Here's how the part is built. I have some questions about the finished solid (model axes, mm). Face numbers are marked on the shaded views. A direction names the side the tool comes from. Give positions to 0.01 mm unless a question says otherwise; leave off trailing zeros. Write each loop counter-clockwise with the first axis right and the second up, starting at its lowest first coordinate (ties: lowest second). Pieces come first, ordered by that corner, then holes. Notation, with made-up numbers: (39.5, 69) - (43.5, 69) arc R35 cw to (43.5, 107) - close; hole circle Ø10 at (11.5, 63.25). An arc over 180 degrees is marked (long way). One line per item, written item: value. Start each with the question number.
1) We'd pull the mould along X, two halves only. Please class the marked faces 4, 5 and 6: +X half, -X half, draft (parallel to the pull), parting line (faces both ways), or undercut.
2) Imagine slicing it at C-C on z = 32. Write out the boundary of the cut face in (x, y), plus the area to 3 significant figures.
3) Please list where these lines run through material, in increasing order: L1, parallel to X at y = 17, z = 4; L2, parallel to Y at x = 91.25, z = 19; L3, parallel to X at y = -4.5, z = 37. Write a range as [from, to].
4) On a 3-axis mill with a long thin cutter (end or side, diameter ignored), from which of +Z, -Z, +X, -X, +Y, -Y can I reach the whole of each face in a straight line? I mean the marked faces 1, 2 and 3. Say none if no direction works.
5) Imagine slicing it at A-A on z = 22. Write out the boundary of the cut face in (x, y), plus the area to 3 significant figures.
6) I'm going to push flat-ended pins straight in: P1, Ø1, axis at x = 97, y = 8, coming from the -Z side; P2, Ø8, axis at y = 8.5, z = 25.5, coming from the +X side (3 decimals); P3, Ø4, axis at y = -4, z = 35, coming from the +X side; P4, Ø1.5, axis at x = 108.8, z = 4, coming from the -Y side. Where does each tip first touch, or does it pass through?
7) Imagine slicing it at D-D on y = 5. Write out the boundary of the cut face in (x, z).
8) Imagine slicing it at B-B on x = 93.3. Write out the boundary of the cut face in (y, z).
from build123d import *

# Parameters (mm, degrees)
SKETCH_2_W          = 20
SKETCH_2_H          = 30
EXTRUDE_1_DEPTH     = 5
SKETCH_5_W          = 20
SKETCH_5_H          = 3
EXTRUDE_3_DEPTH     = 43.51
CUT_EXTRUDE_2_REACH = 125.027
SKETCH_6_W          = 5
SKETCH_6_H          = 13.035
EXTRUDE_4_DEPTH     = 3
CUT_EXTRUDE_3_REACH = 127.702
SKETCH_8_R          = 1.25
CUT_EXTRUDE_4_REACH = 127.702
SKETCH_9_R          = 1.25
CHAMFER_2_SIZE      = 8
CHAMFER_3_SIZE      = 11
EXTRUDE_6_DEPTH     = 3


with BuildPart() as part:
    # 草图2 → 凸台-拉伸1 (new body)
    with BuildSketch(Plane.XY.offset(38.51)):
        with Locations((99.3, 0)):
            Rectangle(SKETCH_2_W, SKETCH_2_H)
        with BuildLine():
            Line((104.3, -3.31662479), (104.3, 3.31662479))
            ThreePointArc((104.3, 3.31662479), (99.3, 6), (94.3, 3.31662479))
            Line((94.3, 3.31662479), (94.3, -3.31662479))
            ThreePointArc((94.3, -3.31662479), (99.3, -6), (104.3, -3.31662479))
        make_face(mode=Mode.SUBTRACT)
    extrude(amount=EXTRUDE_1_DEPTH)

    # 草图5 → 凸台-拉伸3 (add)
    with BuildSketch(Plane.XY.offset(43.51)):
        with Locations((99.3, 16.5)):
            Rectangle(SKETCH_5_W, SKETCH_5_H)
        with Locations((99.3, -16.5)):
            Rectangle(SKETCH_5_W, SKETCH_5_H)
    extrude(amount=-EXTRUDE_3_DEPTH)

    # 草图6 → 切除-拉伸2 (cut, up to next)
    with BuildSketch(Plane.XZ.offset(18), mode=Mode.PRIVATE) as cut_extrude_2_sk1:
        with Locations((102.329663749, 6.5175)):
            Rectangle(SKETCH_6_W, SKETCH_6_H)
    cut_extrude_2_tool1 = extrude(cut_extrude_2_sk1.sketch, amount=-CUT_EXTRUDE_2_REACH, mode=Mode.PRIVATE) & part.part
    add(cut_extrude_2_tool1.solids().sort_by_distance((102.329664, -18, 6.5175))[0], mode=Mode.SUBTRACT)

    # 草图7 → 凸台-拉伸4 (add)
    with BuildSketch(Plane.XZ.offset(18)):
        Polygon((109.3, 10), (112.302663002, 6.997336998), (112.302663002, 0), (109.3, 0), align=None)
    extrude(amount=-EXTRUDE_4_DEPTH)

    # 草图8 → 切除-拉伸3 (cut, up to next)
    with BuildSketch(Plane.XZ.offset(18), mode=Mode.PRIVATE) as cut_extrude_3_sk1:
        with Locations(Location((93.3, 4, 0), (0, 0, 270))):
            Circle(SKETCH_8_R)
    cut_extrude_3_tool1 = extrude(cut_extrude_3_sk1.sketch, amount=-CUT_EXTRUDE_3_REACH, mode=Mode.PRIVATE) & part.part
    # 草图8 → 切除-拉伸3 (cut, up to next)
    with BuildSketch(Plane.XZ.offset(18), mode=Mode.PRIVATE) as cut_extrude_3_sk2:
        with Locations(Location((108.802663002, 4, 0), (0, 0, 270))):
            Circle(SKETCH_8_R)
    cut_extrude_3_tool2 = extrude(cut_extrude_3_sk2.sketch, amount=-CUT_EXTRUDE_3_REACH, mode=Mode.PRIVATE) & part.part
    add(cut_extrude_3_tool1.solids().sort_by_distance((93.3, -18, 4))[0], mode=Mode.SUBTRACT)
    add(cut_extrude_3_tool2.solids().sort_by_distance((108.802663, -18, 4))[0], mode=Mode.SUBTRACT)

    # 草图9 → 切除-拉伸4 (cut, up to next)
    with BuildSketch(Plane(origin=(0, 18, 0), x_dir=(1, 0, 0), z_dir=(0, 1, 0)), mode=Mode.PRIVATE) as cut_extrude_4_sk1:
        with Locations(Location((105.3, -4, 0), (0, 0, 270))):
            Circle(SKETCH_9_R)
    cut_extrude_4_tool1 = extrude(cut_extrude_4_sk1.sketch, amount=-CUT_EXTRUDE_4_REACH, mode=Mode.PRIVATE) & part.part
    # 草图9 → 切除-拉伸4 (cut, up to next)
    with BuildSketch(Plane(origin=(0, 18, 0), x_dir=(1, 0, 0), z_dir=(0, 1, 0)), mode=Mode.PRIVATE) as cut_extrude_4_sk2:
        with Locations(Location((93.3, -4, 0), (0, 0, 90))):
            Circle(SKETCH_9_R)
    cut_extrude_4_tool2 = extrude(cut_extrude_4_sk2.sketch, amount=-CUT_EXTRUDE_4_REACH, mode=Mode.PRIVATE) & part.part
    add(cut_extrude_4_tool1.solids().sort_by_distance((105.3, 18, 4))[0], mode=Mode.SUBTRACT)
    add(cut_extrude_4_tool2.solids().sort_by_distance((93.3, 18, 4))[0], mode=Mode.SUBTRACT)

    # 倒角2
    chamfer_2_edges = [part.edges().sort_by_distance(p)[0] for p in [
        (99.3, -15, 38.51),
        (99.3, 15, 38.51),
    ]]
    chamfer(chamfer_2_edges, length=CHAMFER_2_SIZE)

    # 倒角3
    chamfer_3_edges = [part.edges().sort_by_distance(p)[0] for p in [
        (99.3, 18, 43.51),
        (99.3, -18, 43.51),
    ]]
    chamfer(chamfer_3_edges, length=CHAMFER_3_SIZE)

    # 草图14 → 凸台-拉伸6 (add)
    with BuildSketch(Plane.ZY.offset(-89.3)):
        Polygon((38.51, -7), (30.51, -15), (30.51, 15), (38.51, 7), align=None)
    extrude_6 = extrude(amount=-EXTRUDE_6_DEPTH)

    # 镜向1: 凸台-拉伸6 across plane
    add(extrude_6.mirror(Plane(origin=(99.3, 0, 0), x_dir=(0, 0, 1), z_dir=(1, 0, 0))))


solid = part.part
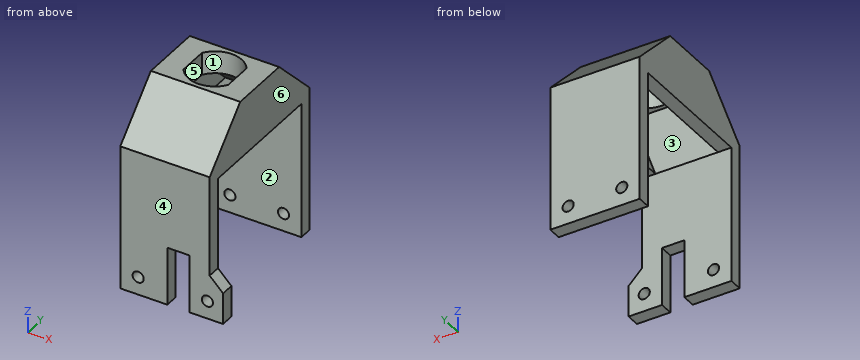
Numbers:
1. face 4: draft
1. face 5: undercut
1. face 6: +X half
2. outline: (89.3, -18) - (109.3, -18) - (109.3, 18) - (89.3, 18) - close; hole (92.3, -13.51) - (106.3, -13.51) - (106.3, 13.51) - (92.3, 13.51) - close
2. area: 342 mm^2
3. L1: [89.3, 92.05], [94.55, 104.05], [106.55, 109.3]
3. L2: [-18, -15], [15, 18]
3. L3: [89.3, 92.3], [106.3, 109.3]
4. face 1: +Z, -Z
4. face 2: -Z, +X, -X
4. face 3: -Z
5. outline: (89.3, -18) - (109.3, -18) - (109.3, -15) - (89.3, -15) - close; (89.3, 15) - (109.3, 15) - (109.3, 18) - (89.3, 18) - close
5. area: 120 mm^2
6. P1: z = 37.01
6. P2: through
6. P3: x = 109.3
6. P4: y = 15
7. outline: (89.3, 30.51) - (92.3, 30.51) - (92.3, 38.51) - (95.98, 38.51) - (95.98, 43.51) - (89.3, 43.51) - close; (102.62, 38.51) - (106.3, 38.51) - (106.3, 30.51) - (109.3, 30.51) - (109.3, 43.51) - (102.62, 43.51) - close
8. outline: (-18, 0) - (-15, 0) - (-15, 2.75) - (-18, 2.75) - close; (-18, 5.25) - (-15, 5.25) - (-15, 30.51) - (-7, 38.51) - (7, 38.51) - (15, 30.51) - (15, 5.25) - (18, 5.25) - (18, 32.51) - (7, 43.51) - (-7, 43.51) - (-18, 32.51) - close; (15, 0) - (18, 0) - (18, 2.75) - (15, 2.75) - close
